from build123d import *

# Parameters (mm, degrees)
SKETCH_1_R      = 1.5
EXTRUDE_4_DEPTH = 3


with BuildPart() as part:
    # 스케치1 → 보스-돌출4 (new body)
    with BuildSketch(Plane.XY):
        Polygon((50, -25), (50, -75), (50, -100), (0, -100), (0, -75), (-50, -75), (-75, -75), (-75, -25), (-50, -25), (-50, 25), (-50, 50), (0, 50), (0, 25), (75, 25), (75, -25), align=None)
        with Locations(Location((70.106183294, -4.68, 0), (0, 0, 180))):
            Circle(SKETCH_1_R, mode=Mode.SUBTRACT)
        with Locations(Location((60.106183294, -4.68, 0), (0, 0, 180))):
            Circle(SKETCH_1_R, mode=Mode.SUBTRACT)
        with Locations(Location((70.106183294, -14.68, 0), (0, 0, 180))):
            Circle(SKETCH_1_R, mode=Mode.SUBTRACT)
        with Locations(Location((60.106183294, -14.68, 0), (0, 0, 180))):
            Circle(SKETCH_1_R, mode=Mode.SUBTRACT)
        with Locations((9.773310691, -85)):
            Circle(SKETCH_1_R, mode=Mode.SUBTRACT)
        with Locations((19.773310691, -85)):
            Circle(SKETCH_1_R, mode=Mode.SUBTRACT)
        with Locations((9.773310691, -95)):
            Circle(SKETCH_1_R, mode=Mode.SUBTRACT)
        with Locations((19.773310691, -95)):
            Circle(SKETCH_1_R, mode=Mode.SUBTRACT)
        with Locations(Location((40.226689309, -95, 0), (0, 0, 180))):
            Circle(SKETCH_1_R, mode=Mode.SUBTRACT)
        with Locations(Location((30.226689309, -95, 0), (0, 0, 180))):
            Circle(SKETCH_1_R, mode=Mode.SUBTRACT)
        with Locations(Location((30.226689309, -85, 0), (0, 0, 180))):
            Circle(SKETCH_1_R, mode=Mode.SUBTRACT)
        with Locations(Location((40.226689309, -85, 0), (0, 0, 180))):
            Circle(SKETCH_1_R, mode=Mode.SUBTRACT)
        with Locations((-39.680330984, 45)):
            Circle(SKETCH_1_R, mode=Mode.SUBTRACT)
        with Locations((-29.680330984, 45)):
            Circle(SKETCH_1_R, mode=Mode.SUBTRACT)
        with Locations((-39.680330984, 35)):
            Circle(SKETCH_1_R, mode=Mode.SUBTRACT)
        with Locations((-29.680330984, 35)):
            Circle(SKETCH_1_R, mode=Mode.SUBTRACT)
        with Locations(Location((-10.319669016, 35, 0), (0, 0, 180))):
            Circle(SKETCH_1_R, mode=Mode.SUBTRACT)
        with Locations(Location((-20.319669016, 35, 0), (0, 0, 180))):
            Circle(SKETCH_1_R, mode=Mode.SUBTRACT)
        with Locations(Location((-20.319669016, 45, 0), (0, 0, 180))):
            Circle(SKETCH_1_R, mode=Mode.SUBTRACT)
        with Locations(Location((-10.319669016, 45, 0), (0, 0, 180))):
            Circle(SKETCH_1_R, mode=Mode.SUBTRACT)
        with Locations(Location((70, 14.68, 0), (0, 0, 180))):
            Circle(SKETCH_1_R, mode=Mode.SUBTRACT)
        with Locations(Location((60, 14.68, 0), (0, 0, 180))):
            Circle(SKETCH_1_R, mode=Mode.SUBTRACT)
        with Locations(Location((70, 4.68, 0), (0, 0, 180))):
            Circle(SKETCH_1_R, mode=Mode.SUBTRACT)
        with Locations(Location((60, 4.68, 0), (0, 0, 180))):
            Circle(SKETCH_1_R, mode=Mode.SUBTRACT)
        with Locations((-70, -35)):
            Circle(SKETCH_1_R, mode=Mode.SUBTRACT)
        with Locations((-60, -35)):
            Circle(SKETCH_1_R, mode=Mode.SUBTRACT)
        with Locations((-70, -45)):
            Circle(SKETCH_1_R, mode=Mode.SUBTRACT)
        with Locations((-60, -45)):
            Circle(SKETCH_1_R, mode=Mode.SUBTRACT)
        with Locations(Location((-60, -55, 0), (0, 0, 180))):
            Circle(SKETCH_1_R, mode=Mode.SUBTRACT)
        with Locations(Location((-70, -55, 0), (0, 0, 180))):
            Circle(SKETCH_1_R, mode=Mode.SUBTRACT)
        with Locations(Location((-60, -65, 0), (0, 0, 180))):
            Circle(SKETCH_1_R, mode=Mode.SUBTRACT)
        with Locations(Location((-70, -65, 0), (0, 0, 180))):
            Circle(SKETCH_1_R, mode=Mode.SUBTRACT)
    extrude(amount=EXTRUDE_4_DEPTH)


solid = part.part
Design review of the part built by this model. Coordinates are the model's own, in mm. Round coordinates to 2 decimals unless told otherwise and drop trailing zeros. Write each loop counter-clockwise with the first axis right and the second up, starting at its lowest first coordinate (ties: lowest second). Pieces come first, ordered by that corner, then holes.
Item 1: Wall thickness on L1, parallel to X at y = -85, z = 1.05; L2, parallel to Y at x = -70, z = 0.75; L3, parallel to Y at x = -9, z = 1.9: over which ranges is each line inside the solid? List them lowest first.
Item 2: For pin 1 Ø1 at (y, z) = (31.5, 1.5) entering from -X; pin 2 Ø1.5 at (x, z) = (-42, 1.5) entering from -Y, all flat-tipped, find the tip position at first contact; note any pin that passes through.
Item 3: Consider section A-A on x = 24.5. Give the boundary of the cut face in (y, z).
Item 4: Consider section B-B on z = 2. Count the separate pieces of the cut face and the enclosed holes in it, and give its area (3 significant figures).
Check values:
1. L1: x = 0 to 8.27, 11.27 to 18.27, 21.27 to 28.73, 31.73 to 38.73, 41.73 to 50
1. L2: y = -75 to -66.5, -63.5 to -56.5, -53.5 to -46.5, -43.5 to -36.5, -33.5 to -25
1. L3: y = -75 to 34.29, 35.71 to 44.29, 45.71 to 50
2. pin 1: stops at x = -50
2. pin 2: stops at y = -75
3. outline: (-100, 0) - (25, 0) - (25, 3) - (-100, 3) - close
4. separate pieces: 1
4. enclosed holes: 32
4. area: 14,800 mm2
